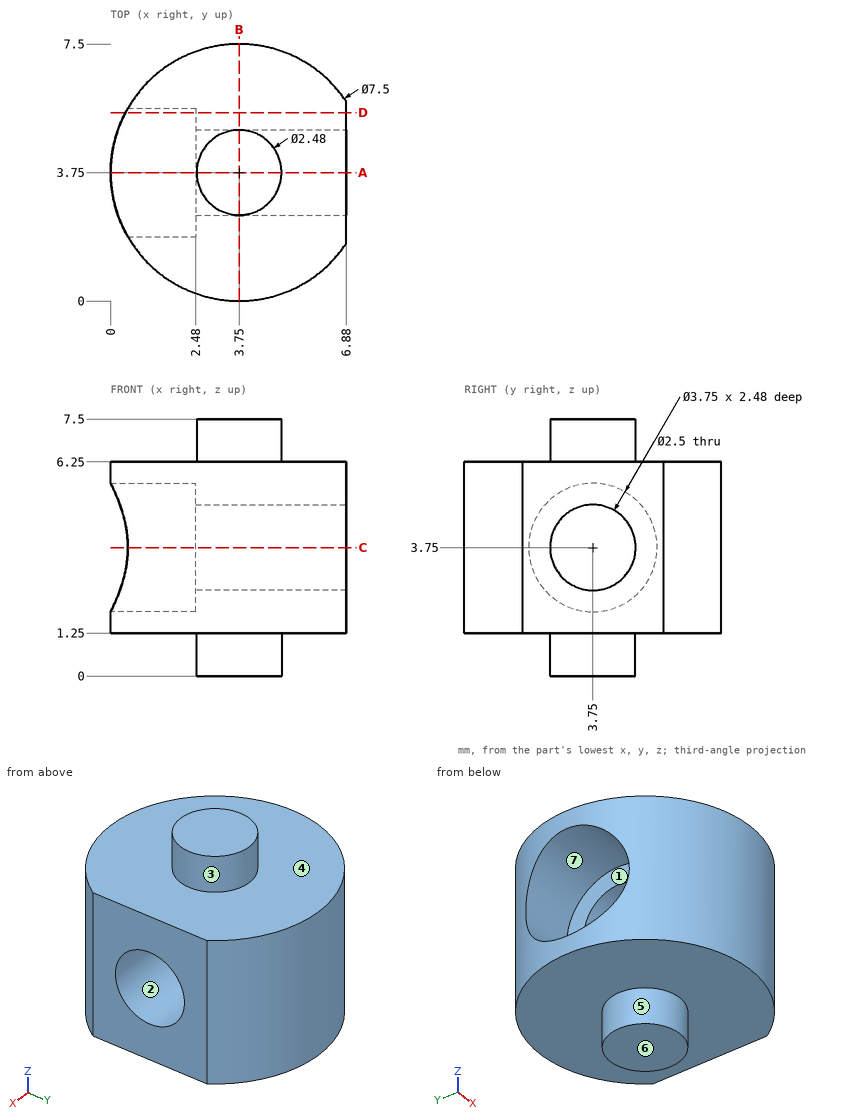
The figure shows three views and two pictorial views of one solid part (mm, origin at its lowest corner). Answer the questions. A direction names the side the tool comes from. Give positions to 0.01 mm unless a question says otherwise; leave off trailing zeros. Write each loop counter-clockwise with the first axis right and the second up, starting at its lowest first coordinate (ties: lowest second). Pieces come first, ordered by that corner, then holes. Notation, with made-up numbers: (89, 54.25) -> (131, 54.25) arc R10 cw to (131, 65.25) -> close; hole circle Ø4 at (84.5, 59.25). An arc over 180 degrees is marked (long way). Use one line per item in the form item = value.
1) Each of these flat-tipped pins is pushed along its axis until it touches: P1, Ø3, axis at y = 3.75, z = 3.75, coming from the -X side; P2, Ø2, axis at x = 1.5, y = 1.5, coming from the -Z side. Where does it stop, or does it pass through?
Result:
P1 = 2.48
P2 = 1.25
2) A tool of negligible diameter and unlimited length cuts with its end or side. For the marked faces 5, 6 and 7, from which of +Z, -Z, +X, -X, +Y, -Y can it reach the whole face along a straight path? Write none if from no direction.
Result:
face_5 = -Z
face_6 = -Z, +X, -X, +Y, -Y
face_7 = -X
3) Straight lines are drawn through the part: probe 1 along Z at (x, y) = (2.5, 7); probe 2 along Y at (x, z) = (5.6, 3.75); probe 3 along Y at (x, z) = (0.75, 3.75) (3 decimals). For each, find the intervals that lie inside material, in ascending order.
Result:
probe_1 = 1.25 to 6.25
probe_2 = 0.49 to 2.5, 5 to 7.01
probe_3 = 1.5 to 1.875, 5.625 to 6
4) Section D-D on y = 5.5 is taken. Write down the section's boundary in (x, z).
Result:
outline = (0.43, 1.25) -> (6.88, 1.25) -> (6.88, 6.25) -> (0.43, 6.25) -> (0.43, 4.42) -> (2.48, 4.42) -> (2.48, 3.08) -> (0.43, 3.08) -> close
5) Section B-B on x = 3.75 is taken. Write down the section's boundary in (y, z), plus the area to 3 significant figures.
Result:
outline = (0, 1.25) -> (2.51, 1.25) -> (2.51, 0) -> (4.99, 0) -> (4.99, 1.25) -> (7.5, 1.25) -> (7.5, 6.25) -> (4.99, 6.25) -> (4.99, 7.5) -> (2.51, 7.5) -> (2.51, 6.25) -> (0, 6.25) -> close; hole circle Ø2.5 at (3.75, 3.75)
area = 38.8 mm²
6) For a pull along Y with two mould halves and no side action, classify the marked faces 1, 2, 3 and 4 as +Y half, -Y half, draft (parallel to the pull), parting line (faces both ways), or undercut.
Result:
face_1 = undercut
face_2 = undercut
face_3 = parting line
face_4 = draft
7) Section C-C on z = 3.75 is taken. Write down the section's boundary in (x, y) (3 decimals), plus the area to 3 significant figures.
Result:
outline = (0.502, 1.875) arc R3.75 ccw to (6.88, 1.685) -> (6.88, 2.5) -> (2.48, 2.5) -> (2.48, 1.875) -> close; (0.502, 5.625) -> (2.48, 5.625) -> (2.48, 5) -> (6.88, 5) -> (6.88, 5.815) arc R3.75 ccw to start
area = 22.8 mm²
8) Section A-A on y = 3.75 is taken. Write down the section's boundary in (x, z) (3 decimals), plus the area to 3 significant figures.
Result:
outline = (0, 1.25) -> (2.51, 1.25) -> (2.51, 0) -> (4.99, 0) -> (4.99, 1.25) -> (6.88, 1.25) -> (6.88, 2.5) -> (2.48, 2.5) -> (2.48, 1.875) -> (0, 1.875) -> close; (0, 5.625) -> (2.48, 5.625) -> (2.48, 5) -> (6.88, 5) -> (6.88, 6.25) -> (4.99, 6.25) -> (4.99, 7.5) -> (2.51, 7.5) -> (2.51, 6.25) -> (0, 6.25) -> close
area = 20.3 mm²
